Here's the drawing with two shaded views (mm, measured from the low corner). I have some questions. A direction names the side the tool comes from. Round coordinates to 2 decimals unless told otherwise and drop trailing zeros. Write each loop counter-clockwise with the first axis right and the second up, starting at its lowest first coordinate (ties: lowest second). Pieces come first, ordered by that corner, then holes. Notation, with made-up numbers: (61, -11) - (105, -11) arc R8 cw to (105, -2) - close; hole circle Ø5 at (-14, 6.25). An arc over 180 degrees is marked (long way). Return JSON: item names as keys, results as strings. Group by question number.
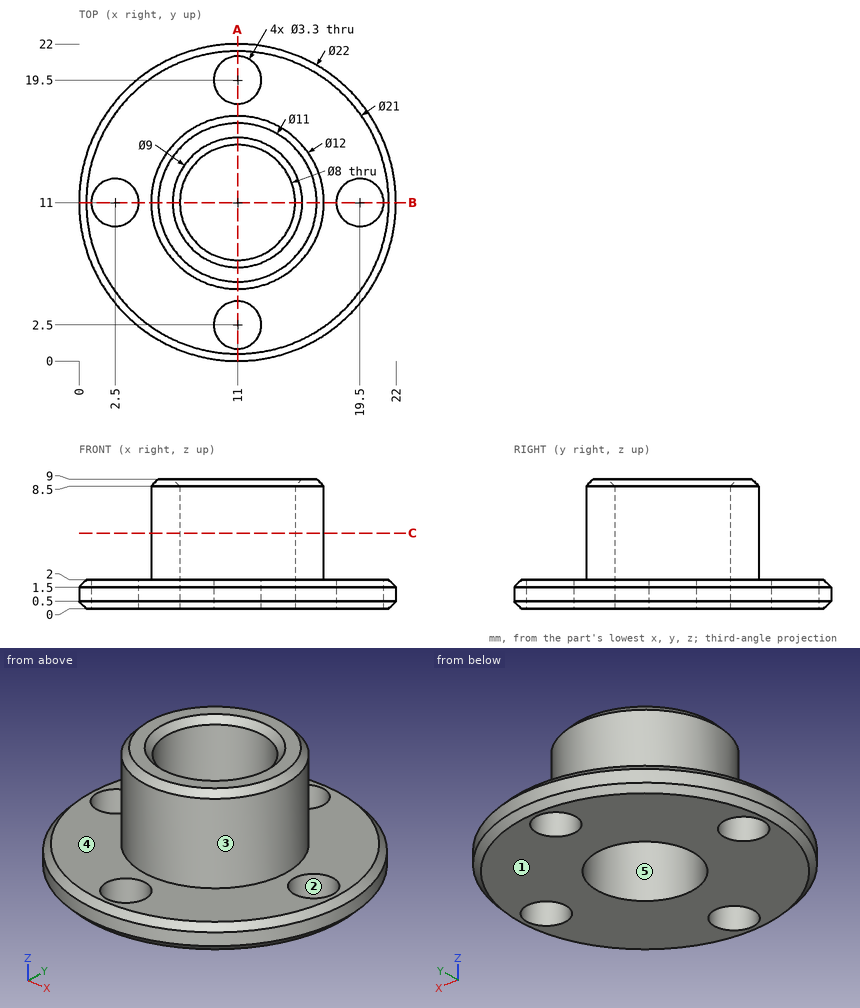
1) Will these pins go through, and if not, where does the flat tip stop? pin 1 Ø4.5 at (x, y) = (11, 2.5) entering from +Z; pin 2 Ø2 at (x, z) = (8, 7) entering from +Y; pin 3 Ø3 at (x, y) = (19.5, 11) entering from +Z; pin 4 Ø1 at (x, y) = (14, 13.5) entering from +Z.
2) Imagine slicing it at A-A (x = 11). Please give me the cut outline in (y, z).
3) If we mould it in two halves opening along X, with no side actions, what happens to the marked faces 1, 2 and 3? For each: released by +X, released by -X, zero draft, split by the parting line, or undercut.
4) For the marked faces 4 and 5, which set-ups out of +Z, -Z, +X, -X, +Y, -Y let a thin tool reach every point of the face, with its end or its side?
5) Imagine slicing it at C-C (z = 5.25). Please give me the cut outline in (x, y).
6) I need wall thicknesses on line 1 along Y through (x, z) = (11, 1.45); line 2 along Y through (x, z) = (11, 6.75); line 3 along Z through (x, y) = (17, 11.75). Which ranges of each line are inside material? Lowest first, please.
Results found:
{
 "1": {"pin 1": "stops at z = 2", "pin 2": "stops at y = 16.66", "pin 3": "passes through", "pin 4": "stops at z = 8.91"},
 "2": {"outline": "(0, 0.5) - (0.5, 0) - (0.85, 0) - (0.85, 2) - (0.5, 2) - (0, 1.5) - close; (4.15, 0) - (7, 0) - (7, 8.5) - (6.5, 9) - (5.5, 9) - (5, 8.5) - (5, 2) - (4.15, 2) - close; (15, 0) - (17.85, 0) - (17.85, 2) - (17, 2) - (17, 8.5) - (16.5, 9) - (15.5, 9) - (15, 8.5) - close; (21.15, 0) - (21.5, 0) - (22, 0.5) - (22, 1.5) - (21.5, 2) - (21.15, 2) - close"},
 "3": {"face 1": "zero draft", "face 2": "undercut", "face 3": "split by the parting line"},
 "4": {"face 4": "+Z", "face 5": "+Z, -Z"},
 "5": {"outline": "circle Ø12 at (11, 11); hole circle Ø8 at (11, 11)"},
 "6": {"line 1": "y = 0 to 0.85, 4.15 to 7, 15 to 17.85, 21.15 to 22", "line 2": "y = 5 to 7, 15 to 17", "line 3": "z = 0 to 2"}
}
